The listing builds one solid part. Answer for the finished solid, in the listing's coordinates (mm). A direction names the side the tool comes from. Give positions to 0.01 mm unless a question says otherwise; leave off trailing zeros. Write each loop counter-clockwise with the first axis right and the second up, starting at its lowest first coordinate (ties: lowest second). Pieces come first, ordered by that corner, then holes. Notation, with made-up numbers: (-25, 13.25) -> (6, 13.25) arc R18 ccw to (6, 39.25) -> close; hole circle Ø1 at (43, 51.5). An arc over 180 degrees is marked (long way). One line per question, with ' | ' between items.
from build123d import *

# Parameters (mm, degrees)
SKETCH1_W           = 275
SKETCH1_H           = 25
SKETCH1_R           = 1.6
BOSS_EXTRUDE1_DEPTH = 6
SKETCH2_W           = 2.5
SKETCH2_H           = 25
BOSS_EXTRUDE2_DEPTH = 5


with BuildPart() as part:
    # Sketch1 → Boss-Extrude1 (new body)
    with BuildSketch(Plane(origin=(0, 0, 0), x_dir=(1, 0, 0), z_dir=(0, 1, 0))):
        Rectangle(SKETCH1_W, SKETCH1_H)
        with Locations(Location((-135, 0, 0), (0, 0, 270))):
            Circle(SKETCH1_R, mode=Mode.SUBTRACT)
        with Locations(Location((132, 0, 0), (0, 0, 270))):
            Circle(SKETCH1_R, mode=Mode.SUBTRACT)
        with Locations(Location((22, 0, 0), (0, 0, 270))):
            Circle(SKETCH1_R, mode=Mode.SUBTRACT)
    extrude(amount=BOSS_EXTRUDE1_DEPTH)

    # Sketch2 → Boss-Extrude2 (add)
    with BuildSketch(Plane(origin=(0, 0, 0), x_dir=(-1, 0, 0), z_dir=(0, -1, 0))):
        with Locations((-136.25, 0)):
            Rectangle(SKETCH2_W, SKETCH2_H)
    extrude(amount=BOSS_EXTRUDE2_DEPTH)


solid = part.part
Item 1: Flat-ended cylindrical pins translate along their axes: pin 1 (4 mm diameter, centred on x = -135, z = 0, fed in from +Y); pin 2 (3 mm diameter, centred on x = -72, z = -5, fed in from -Y). Find the tip coordinate at first contact, or state that the pin passes through.
Answers below:
pin 1: y = 6 | pin 2: y = 0
Item 2: Consider line 1 (X direction, y = 2.25, z = 0.25); line 2 (Z direction, x = 132, y = 2.4); line 3 (Y direction, x = -90, z = -3.75). Determine where each line is inside the solid, lowest interval first. Write a range as [from, to].
Answers below:
line 1: [-137.5, -136.58], [-133.42, 20.42], [23.58, 130.42], [133.58, 137.5] | line 2: [-12.5, -1.6], [1.6, 12.5] | line 3: [0, 6]
Item 3: Find section A-A (z = -4). Write down the section's boundary in (x, y).
Answers below:
outline: (-137.5, 0) -> (135, 0) -> (135, -5) -> (137.5, -5) -> (137.5, 6) -> (-137.5, 6) -> close
Item 4: A tool of negligible diameter and unlimited length cuts with its end or side. For faces 1 (the face through (137.5, 1, 0)), 2 (the face through (-3, 0, 0)), from which of +Z, -Z, +X, -X, +Y, -Y can it reach the whole face along a straight path? Write none if from no direction.
Answers below:
face 1: +Z, -Z, +X, +Y, -Y | face 2: +Z, -Z, -X, -Y
Item 5: Find section B-B (x = 96). Write down the section's boundary in (y, z), then the cut area to 3 significant figures.
Answers below:
outline: (0, -12.5) -> (6, -12.5) -> (6, 12.5) -> (0, 12.5) -> close | area: 150 mm²
